```python
from build123d import *

# Parameters (mm, degrees)
SKETCH1_W               = 22.25
SKETCH1_H               = 5
BOSS_EXTRUDE1_DEPTH     = 10
FILLET2_R               = 9
FILLET4_R               = 30
SKETCH4_R               = 4.25
CUT_EXTRUDE1_DEPTH      = 74
CUT_EXTRUDE3_DEPTH      = 45.497893381
CUT_EXTRUDE3_DEPTH_BACK = 45.497893381
SKETCH6_R               = 1.5
SKETCH7_R               = 5
SKETCH7_R_2             = 3.25
BOSS_EXTRUDE2_DEPTH     = 5
FILLET6_R               = 1
CUT_EXTRUDE4_DEPTH      = 45.497893381
CUT_EXTRUDE4_DEPTH_BACK = 45.497893381
SKETCH8_R               = 1.5


with BuildPart() as part:
    # Sketch1 → Revolve1 (revolve)
    with BuildSketch(Plane.XY):
        Polygon((25.5, -22.75), (25.5, -12.75), (9.85, -12.75), (9.85, -18.75), (0, -18.75), (0, -22.75), align=None)
        with Locations((14.375, 15.25)):
            Rectangle(SKETCH1_W, SKETCH1_H)
    revolve(axis=Axis((0, -12.75, 0), (0, 1, 0)))


with BuildPart() as body_2:
    # Sketch2 → Boss-Extrude1 (new, symmetric)
    with BuildSketch(Plane.XY):
        Polygon((25.5, -22.75), (28.5, -22.75), (28.5, 17.75), (25.5, 17.75), (20.5, 17.75), (20.5, -22.75), align=None)
    extrude(amount=BOSS_EXTRUDE1_DEPTH, both=True)


with BuildPart() as part_1:
    add(part.part)

    # Intersect2: read off the stored shape, not the designer's step
    # Intersect2: union body 2
    add(body_2.part)

    # Fillet2
    # the kernel refuses this fillet: 9 mm, written as the material it takes off along each edge
    with BuildSketch(Plane(origin=(28.5, -45.110679775, -10), x_dir=(-1, 0, 0), z_dir=(0, 1, 0))) as fillet2_piece_1_section:
        with BuildLine():
            CenterArc((9, 8.94427191), FILLET2_R, 180, 83.620629792)
            Line((0, 8.94427191), (0, 0))
            Line((0, 0), (8, 0))
        make_face()
    fillet2_piece_1 = extrude(amount=85.22135955, mode=Mode.PRIVATE)
    fillet2_piece_1 = fillet2_piece_1 - Plane(origin=(0, -45.110679775, 0), x_dir=(1, 0, 0), z_dir=(0, 1, 0)) * Cylinder(25.5, 207, mode=Mode.PRIVATE)
    add(fillet2_piece_1, mode=Mode.SUBTRACT)
    with BuildSketch(Plane(origin=(28.5, -45.110679775, -10), x_dir=(-1, 0, 0), z_dir=(0, 1, 0))) as fillet2_piece_2_section:
        with BuildLine():
            CenterArc((9, 8.94427191), FILLET2_R, 180, 83.620629792)
            Line((0, 8.94427191), (0, 0))
            Line((0, 0), (8, 0))
        make_face()
    fillet2_piece_2 = extrude(amount=85.22135955, mode=Mode.PRIVATE)
    fillet2_piece_2 = split(fillet2_piece_2, bisect_by=Plane(origin=(28.5, -12.75, -10), z_dir=(0, 1, 0)), keep=Keep.TOP, mode=Mode.PRIVATE)
    fillet2_piece_2 = split(fillet2_piece_2, bisect_by=Plane(origin=(28.5, 12.75, -10), z_dir=(0, -1, 0)), keep=Keep.TOP, mode=Mode.PRIVATE)
    add(fillet2_piece_2, mode=Mode.SUBTRACT)
    with BuildSketch(Plane(origin=(28.5, -45.110679775, 10), x_dir=(-1, 0, 0), z_dir=(0, 1, 0))) as fillet2_piece_3_section:
        with BuildLine():
            CenterArc((9, -8.94427191), FILLET2_R, 96.379370208, 83.620629792)
            Line((0, -8.94427191), (0, 0))
            Line((0, 0), (8, 0))
        make_face()
    fillet2_piece_3 = extrude(amount=85.22135955, mode=Mode.PRIVATE)
    fillet2_piece_3 = fillet2_piece_3 - Plane(origin=(0, -45.110679775, 0), x_dir=(1, 0, 0), z_dir=(0, 1, 0)) * Cylinder(25.5, 207, mode=Mode.PRIVATE)
    add(fillet2_piece_3, mode=Mode.SUBTRACT)
    with BuildSketch(Plane(origin=(28.5, -45.110679775, 10), x_dir=(-1, 0, 0), z_dir=(0, 1, 0))) as fillet2_piece_4_section:
        with BuildLine():
            CenterArc((9, -8.94427191), FILLET2_R, 96.379370208, 83.620629792)
            Line((0, -8.94427191), (0, 0))
            Line((0, 0), (8, 0))
        make_face()
    fillet2_piece_4 = extrude(amount=85.22135955, mode=Mode.PRIVATE)
    fillet2_piece_4 = split(fillet2_piece_4, bisect_by=Plane(origin=(28.5, -12.75, 10), z_dir=(0, 1, 0)), keep=Keep.TOP, mode=Mode.PRIVATE)
    fillet2_piece_4 = split(fillet2_piece_4, bisect_by=Plane(origin=(28.5, 12.75, 10), z_dir=(0, -1, 0)), keep=Keep.TOP, mode=Mode.PRIVATE)
    add(fillet2_piece_4, mode=Mode.SUBTRACT)

    # Fillet4
    fillet4_edges = [part_1.edges().sort_by_distance(p)[0] for p in [
        (23.892282884, 15.25, -8.911162582),
        (23.892282884, -17.75, -8.911162582),
        (23.892282884, 15.25, 8.911162582),
        (23.892282884, -17.75, 8.911162582),
    ]]
    fillet(fillet4_edges, radius=FILLET4_R)

    # Sketch4 → Cut-Extrude1 (cut)
    with BuildSketch(Plane(origin=(0, 0, 0), x_dir=(0, 0, -1), z_dir=(1, 0, 0))):
        with Locations(Location((0, 0, 0), (0, 0, 255.616756445))):
            Circle(SKETCH4_R)
    extrude(amount=CUT_EXTRUDE1_DEPTH, mode=Mode.SUBTRACT)

    # Sketch6 → Cut-Extrude3 (cut, two sides: drawn at the far end of the back side and taken through both)
    with BuildSketch(Plane.XY.offset(-CUT_EXTRUDE3_DEPTH_BACK)):
        with Locations((24.798321038, 0)):
            Circle(SKETCH6_R)
    extrude(amount=CUT_EXTRUDE3_DEPTH + CUT_EXTRUDE3_DEPTH_BACK, mode=Mode.SUBTRACT)

    # Sketch7 → Boss-Extrude2 (add)
    with BuildSketch(Plane(origin=(0, 17.75, 0), x_dir=(1, 0, 0), z_dir=(0, 1, 0))):
        Circle(SKETCH7_R)
        Circle(SKETCH7_R_2, mode=Mode.SUBTRACT)
    extrude(amount=BOSS_EXTRUDE2_DEPTH)

    # Fillet6
    fillet6_edges = [part_1.edges().sort_by_distance(p)[0] for p in [
        (-5, 17.75, 0),
    ]]
    fillet(fillet6_edges, radius=FILLET6_R)

    # Sketch8 → Cut-Extrude4 (cut, two sides: drawn at the far end of the back side and taken through both)
    with BuildSketch(Plane.XY.offset(-CUT_EXTRUDE4_DEPTH_BACK)):
        with Locations((0, 20.25)):
            Circle(SKETCH8_R)
    extrude(amount=CUT_EXTRUDE4_DEPTH + CUT_EXTRUDE4_DEPTH_BACK, mode=Mode.SUBTRACT)


solid = part_1.part
```
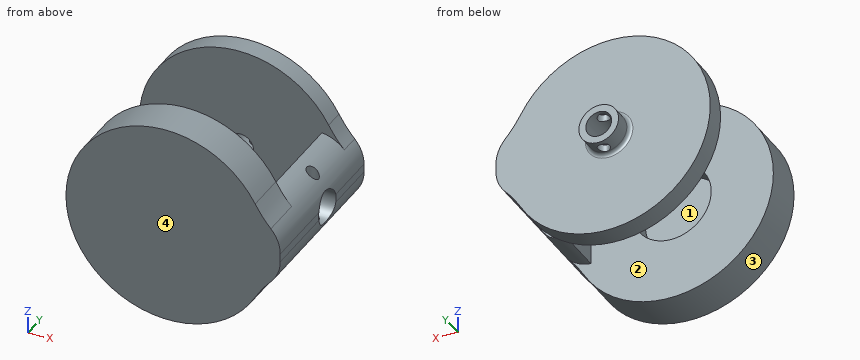
Input: part model. Units: mm. Frame: model coordinates. Face numbers are marked on the shaded views. Coordinates: 2 decimals unless noted, no trailing zeros. Loops run counter-clockwise (first coordinate to the right, second up) from the corner with the lowest first, then second, coordinate; pieces in that order, holes last. Notation, with made-up numbers: M 49,18 L 97,18 A22 cw 97,24 Z; hole C 55.25,-39.75 d1. An arc over 180 degrees is marked long. Answer in a Markdown table with one row per item.
1. Section C-C, the plane y = 20.25. Output: boundary loops of the cut face in (x, z), then the cut area to 3 significant figures.
Response:
| item | result |
|---|---|
| outline | M -1.5,-4.77 L -1.5,-2.88 A3.25 cw -1.5,2.88 L -1.5,4.77 A5 ccw Z; M 1.5,-4.77 A5 ccw 1.5,4.77 L 1.5,2.88 A3.25 cw 1.5,-2.88 Z |
| area | 34.6 mm2 |
2. Section D-D, the plane y = 0. Output: boundary loops of the cut face in (x, z).
Response:
| item | result |
|---|---|
| outline | M 20.5,-10 A9 ccw 23.3,-9.21 L 23.3,-4.25 L 20.5,-4.25 Z; M 20.5,4.25 L 23.3,4.25 L 23.3,9.21 A9 ccw 20.5,10 Z; M 26.3,-6.95 A9 ccw 27.91,-4.25 L 26.3,-4.25 Z; M 26.3,4.25 L 27.91,4.25 A9 ccw 26.3,6.95 Z |
3. Material intervals for line 1 (Y direction, x = 0, z = 3.6); line 2 (Y direction, x = -4, z = 2); line 3 (Y direction, x = -11, z = 17), sorted ascending.
Response:
| item | result |
|---|---|
| line 1 | y = -22.75 to -18.75, 12.75 to 18.75, 21.75 to 22.75 |
| line 2 | y = -22.75 to -18.75, 12.75 to 22.75 |
| line 3 | y = -22.75 to -12.75, 12.75 to 17.75 |
4. Section B-B, the plane x = -14. Output: boundary loops of the cut face in (y, z).
Response:
| item | result |
|---|---|
| outline | M -22.75,-21.31 L -12.75,-21.31 L -12.75,21.31 L -22.75,21.31 Z; M 12.75,-21.31 L 17.75,-21.31 L 17.75,21.31 L 12.75,21.31 Z |
5. Section A-A, the plane z = 0. Output: boundary loops of the cut face in (x, y).
Response:
| item | result |
|---|---|
| outline | M -25.5,-22.75 L 28.5,-22.75 L 28.5,-4.25 L 20.5,-4.25 L 20.5,-12.75 L 9.85,-12.75 L 9.85,-18.75 L -9.85,-18.75 L -9.85,-12.75 L -25.5,-12.75 Z; M -25.5,12.75 L -3.25,12.75 L -3.25,22.75 L -5,22.75 L -5,18.75 A1 cw -6,17.75 L -25.5,17.75 Z; M 3.25,12.75 L 20.5,12.75 L 20.5,4.25 L 28.5,4.25 L 28.5,17.75 L 6,17.75 A1 cw 5,18.75 L 5,22.75 L 3.25,22.75 Z |
6. First-contact query: pin 1 (3.5 mm diameter, centred on x = 0, y = 20.25, fed in from -Z); pin 2 (10 mm diameter, centred on x = 14, y = 10.5, fed in from +Z); pin 3 (2 mm diameter, centred on x = -10, y = -10, fed in from -Z); pin 4 (1.5 mm diameter, centred on y = 16.5, z = -13, fed in from -X). Flat tips, straight axial feed; report the tip coordinate or a pass-through.
Response:
| item | result |
|---|---|
| pin 1 | stops at z = -5.03 |
| pin 2 | stops at z = 23.65 |
| pin 3 | passes through |
| pin 4 | stops at x = -22.36 |
7. Draft query along Y for the marked faces 1, 2, 3 and 4. Return one class per face: pulls with the +Y half, pulls with the -Y half, needs draft (parallel to the pull), parting line crosses it, or undercut.
Response:
| item | result |
|---|---|
| face 1 | undercut |
| face 2 | undercut |
| face 3 | needs draft |
| face 4 | pulls with the -Y half |
